The model under review builds one solid part; all positions refer to its coordinate system, in mm. Round coordinates to 2 decimals unless told otherwise and drop trailing zeros.
from build123d import *

# Parameters (mm, degrees)
BOSS_EXTRUDE1_DEPTH    = 4
FILLET1_R              = 2
F_8_0MM_DOWEL_HOLE1_D  = 8
M20X1_5_TAPPED_HOLE1_D = 18.5


with BuildPart() as part:
    # Sketch1 → Boss-Extrude1 (new body)
    with BuildSketch(Plane(origin=(0, 0, 0), x_dir=(1, 0, 0), z_dir=(0, 1, 0))):
        with BuildLine():
            Line((-90.571428571, 63.839285714), (109.428571429, 63.839285714))
            ThreePointArc((109.428571429, 63.839285714), (116.49963924, 60.910353526), (119.428571429, 53.839285714))
            Line((119.428571429, 53.839285714), (119.428571429, -51.160714286))
            ThreePointArc((119.428571429, -51.160714286), (116.49963924, -58.231782098), (109.428571429, -61.160714286))
            Line((109.428571429, -61.160714286), (-90.571428571, -61.160714286))
            ThreePointArc((-90.571428571, -61.160714286), (-97.642496383, -58.231782098), (-100.571428571, -51.160714286))
            Line((-100.571428571, -51.160714286), (-100.571428571, 53.839285714))
            ThreePointArc((-100.571428571, 53.839285714), (-97.642496383, 60.910353526), (-90.571428571, 63.839285714))
        make_face()
    extrude(amount=BOSS_EXTRUDE1_DEPTH)

    # Fillet1
    fillet1_edges = [part.edges().sort_by_distance(p)[0] for p in [
        (-97.642496383, 4, -60.910353526),
        (-100.571428571, 4, -1.339285714),
        (-97.642496383, 4, 58.231782098),
        (9.428571429, 4, 61.160714286),
        (116.49963924, 4, 58.231782098),
        (119.428571429, 4, -1.339285714),
        (116.49963924, 4, -60.910353526),
        (9.428571429, 4, -63.839285714),
    ]]
    fillet(fillet1_edges, radius=FILLET1_R)

    # Ø8.0mm Dowel Hole1 (through all)
    with Locations(Plane(origin=(0, 4, 0), x_dir=(1, 0, 0), z_dir=(0, 1, 0))):
        with Locations((-90.571428571, 53.839285714), (109.428571429, 53.839285714), (-90.571428571, -51.160714286), (109.428571429, -51.160714286), (109.428571429, 1.339285714), (9.428571429, 53.839285714), (-90.571428571, 1.339285714), (9.428571429, -51.160714286)):
            Hole(F_8_0MM_DOWEL_HOLE1_D / 2)

    # M20x1.5 Tapped Hole1 (through all)
    with Locations(Plane(origin=(0, 4, 0), x_dir=(1, 0, 0), z_dir=(0, 1, 0))):
        with Locations((-20.571428571, 1.339285714)):
            Hole(M20X1_5_TAPPED_HOLE1_D / 2)


solid = part.part
(1) Clearance check with a flat-ended pin moving along its axis: P1, Ø6.5, axis at x = 9.43, z = -53.84, coming from the +Y side. State where the tip first meets the part, or that it passes through.
(2) To check wall thickness, follow L1, parallel to Z at x = 11, y = 2.95; L2, parallel to Z at x = 12, y = 2.15; L3, parallel to Z at x = -88.5, y = 1.15. State the ranges of each line that lie inside material, in increasing order.
(3) We need section A-A (y = 3.1). Count the separate pieces of the cut face and the enclosed holes in it, and give its area (3 significant figures).
(4) The part is to be moulded in two halves that separate along Z. For faces 1 (the cylindrical face through (116.58, 0.99, 58.15)), 2 (the cylindrical face through (-94.4, 2, -2.5)), 3 (the cylindrical face through (-97.72, 0.99, -60.83)), 4 (the cylindrical face through (-94.266, 1.972, 52.693)), say which applies: pulls with the +Z half, pulls with the -Z half, needs draft (parallel to the pull), parting line crosses it, or undercut.
Verdict:
1. P1: passes through
2. L1: z = -63.6 to -57.52, -50.16 to 47.48, 54.84 to 60.92
2. L2: z = -63.83 to -56.9, -50.78 to 48.1, 54.22 to 61.16
2. L3: z = -63.84 to -57.26, -50.42 to -4.76, 2.08 to 47.74, 54.58 to 61.16
3. separate pieces: 1
3. enclosed holes: 9
3. area: 26,500 mm2
4. face 1: pulls with the +Z half
4. face 2: undercut
4. face 3: pulls with the -Z half
4. face 4: undercut
